Autodesk Inventor part; units mm, degrees
ref_plane "YZ Plane" through (0, 0, 0) normal (1, 0, 0) x (0, 1, 0)
ref_plane "XZ Plane" through (0, 0, 0) normal (0, 1, 0) x (-1, 0, 0)
ref_plane "XY Plane" through (0, 0, 0) normal (0, 0, 1) x (1, 0, 0)
sketch "Sketch1" plane through (0, 0, 0) normal (0, 0, 1) x (1, 0, 0)
  line L0 (-20, 3) -> (96, 3) construction
  line L1 (-20, -2) -> (96, -2)
  line L2 (96, 8) -> (-20, 8)
  arc A0 (-20, 8) -> (-20, -2) centre (-20, 3) ccw
  arc A1 (96, -2) -> (96, 8) centre (96, 3) ccw
  circle A2 centre (-20, 3) radius 2.5
  circle A3 centre (96, 3) radius 2.5
  point P0 (0, 0)
  point P1 (38, 3)
  dimension "d0" = 10
  dimension "d1" = 5
  dimension "d2" = 116
extrude "Extrusion1" add sketch "Sketch1" along normal blind 5 contours A0 L2 A1 L1 | A3
extrude "Extrusion2" add sketch "Sketch1" against normal blind 5 contours A3
properties material "Copper, Alloy"
Design review of the part built by this model. Coordinates are the model's own, in mm. A direction names the side the tool comes from. Coordinates: 2 decimals unless noted, no trailing zeros. Loops run counter-clockwise (first coordinate to the right, second up) from the corner with the lowest first, then second, coordinate; pieces in that order, holes last.
Item 1: Clearance check with flat-ended pins moving along their axes: pin 1 (4 mm diameter, centred on x = -20, y = 3, fed in from +Z); pin 2 (1 mm diameter, centred on y = 7, z = 0, fed in from +X); pin 3 (5 mm diameter, centred on x = 61, y = 2, fed in from -Z); pin 4 (2 mm diameter, centred on y = 4.5, z = 4, fed in from -X). State where each tip first meets the part, or that it passes through.
Completed:
pin 1: passes through
pin 2: stops at x = 99.57
pin 3: stops at z = 0
pin 4: stops at x = -24.97
Item 2: Add section A-A (y = 3). Write out the cut boundary in (x, z), and give its area (3 significant figures).
Completed:
outline: (-25, 0) - (-22.5, 0) - (-22.5, 5) - (-25, 5) - close; (-17.5, 0) - (93.5, 0) - (93.5, -5) - (98.5, -5) - (98.5, 0) - (101, 0) - (101, 5) - (-17.5, 5) - close
area: 630 mm2
Item 3: Draft analysis for pull direction Y (two halves, no side actions). For faces 3 (the flat face through (37, 3, 0)), 4 (the cylindrical face through (-25, 3, 2)), 5 (the flat face through (37, -2, 2)), 6 (the cylindrical face through (-22.5, 2.9, 2.5)), state which applies: pulls with the +Y half, pulls with the -Y half, needs draft (parallel to the pull), parting line crosses it, or undercut.
Completed:
face 3: needs draft
face 4: parting line crosses it
face 5: pulls with the -Y half
face 6: undercut
Item 4: Add section B-B (x = -14). Write out the cut boundary in (y, z).
Completed:
outline: (-2, 0) - (8, 0) - (8, 5) - (-2, 5) - close
Item 5: For faces 1 (the flat face through (96, 3, -5)), 2 (the cylindrical face through (94, 1.5, -2.5)), list the 3-axis set-ups (+Z, -Z, +X, -X, +Y, -Y) from which the entire face can be reached by the end or side of a thin tool; tool diameter is ignored.
Completed:
face 1: -Z, +X, -X, +Y, -Y
face 2: -Z
Item 6: Add section C-C (z = -1.75). Write out the cut boundary in (x, y), and give its area (3 significant figures).
Completed:
outline: circle Ø5 at (96, 3)
area: 19.6 mm2
Item 7: Wall thickness on L1, parallel to Z at x = 49.5, y = 2.75; L2, parallel to Y at x = -20, z = 2.25; L3, parallel to X at y = 2.25, z = -3.5: over which ranges is each line inside the solid? List them lowest first.
Completed:
L1: z = 0 to 5
L2: y = -2 to 0.5, 5.5 to 8
L3: x = 93.62 to 98.38
